Job drawing, mm, ordinate dimensions from the low corner. One solid piece. Coordinates: 2 decimals unless noted, no trailing zeros. Loops run counter-clockwise (first coordinate to the right, second up) from the corner with the lowest first, then second, coordinate; pieces in that order, holes last. Notation, with made-up numbers: M 89.5,74 L 105.5,74 A30 ccw 105.5,97 Z; hole C -21.5,-37 d2. An arc over 180 degrees is marked long. Answer as a JSON object with one key per item and string values. Group by question number.
1. Saw through at B-B on x = 50. Write the cut outline in (y, z), then the cut area to 3 significant figures.
2. Saw through at A-A on z = 12.5. Write the cut outline in (x, y).
3. Saw through at C-C on y = 1.65. Write the cut outline in (x, z), then the cut area to 3 significant figures.
4. Drill centre lines: L1, parallel to Z at x = 50, y = 1.15; L2, parallel to X at y = 0.6, z = 12.5; L3, parallel to X at y = 1.25, z = 15.25. Where is each one in solid material? Low to high.
5. Drop a flat-ended pin along its axis: pin 1 Ø5 at (x, z) = (37, 8) entering from -Y. Give the stop position or say it passes through.
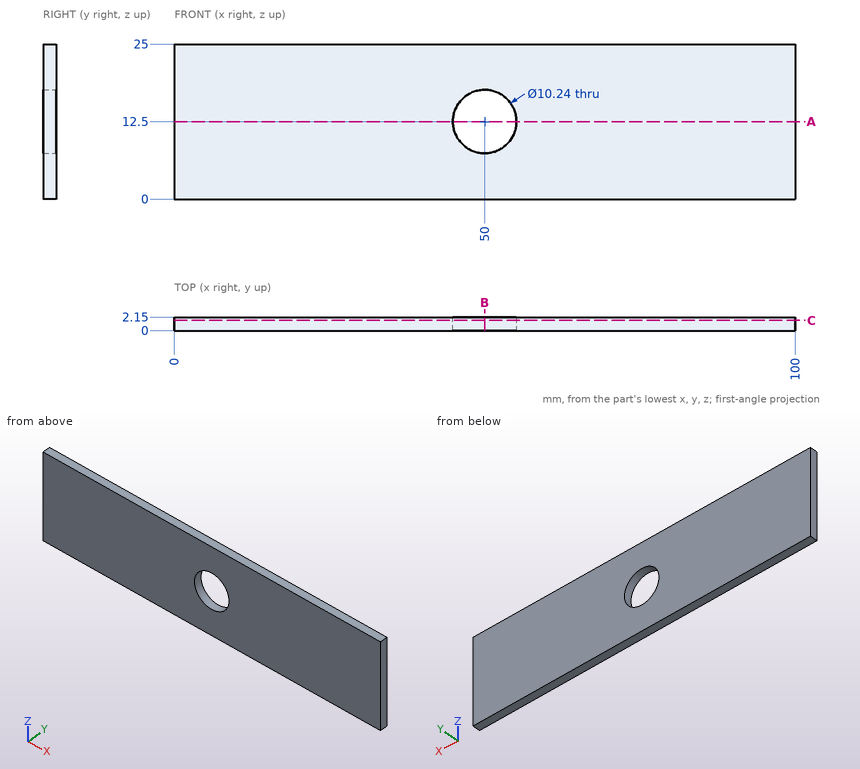
Outcome:
{
 "1": {"outline": "M 0,0 L 2.15,0 L 2.15,7.38 L 0,7.38 Z; M 0,17.62 L 2.15,17.62 L 2.15,25 L 0,25 Z", "area": "31.7 mm²"},
 "2": {"outline": "M 0,0 L 44.88,0 L 44.88,2.15 L 0,2.15 Z; M 55.12,0 L 100,0 L 100,2.15 L 55.12,2.15 Z"},
 "3": {"outline": "M 0,0 L 100,0 L 100,25 L 0,25 Z; hole C 50,12.5 d10.24", "area": "2,420 mm²"},
 "4": {"L1": "z = 0 to 7.38, 17.62 to 25", "L2": "x = 0 to 44.88, 55.12 to 100", "L3": "x = 0 to 45.68, 54.32 to 100"},
 "5": {"pin 1": "stops at y = 0"}
}
